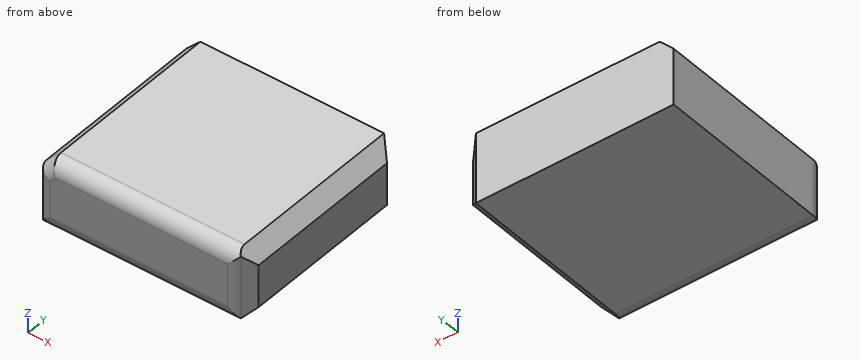
```python
from build123d import *

# Parameters (mm, degrees)
F0_W        = 76.2943662703
F0_H        = 68.5328170657
F1_DEPTH    = 25.4
F2_SIZE     = 5.08
F3_T1_DEPTH = 45.72
F3_T3_DEPTH = 32.5842048969
F3_T5_DEPTH = 96.6143662703
F3_T7_DEPTH = 91.5343662703
F3_T9_DEPTH = 35.9210244843


# Not quite as in the source:
# - a fillet or chamfer that OpenCascade refuses, or shapes differently, is made with other operations: its cross-section is extruded or revolved along the edge and cut away or added


with BuildPart() as f1:
    # F0 (on Top) → F1 (new body)
    with BuildSketch(Plane.XY):
        with Locations((-1.9816737622, 2.3119486868)):
            Rectangle(F0_W, F0_H)
    extrude(amount=F1_DEPTH)

    # F2
    f2_edges = [f1.edges().sort_by_distance(p)[0] for p in [
        (36.165509, -31.95446, 12.7),
        (36.165509, 36.578357, 12.7),
        (36.165509, 2.311949, 0),
        (36.165509, 2.311949, 25.4),
        (-40.128857, 2.311949, 25.4),
    ]]
    chamfer(f2_edges, length=F2_SIZE)

    # F3: fillet of radius 5.08 on 5 edges, made by hand

    # F3_s2 → F3_t1 (cut)
    with BuildSketch(Plane.XY.offset(-12.7)):
        with BuildLine():
            ThreePointArc((-40.1288568974, -26.874459846), (-38.6409593458, -30.4665622944), (-35.0488568974, -31.954459846))
            Line((-35.0488568974, -31.954459846), (-40.1288568974, -31.954459846))
            Line((-40.1288568974, -31.954459846), (-40.1288568974, -26.874459846))
        make_face()
    extrude(amount=F3_T1_DEPTH, mode=Mode.SUBTRACT)

    # F3_s4 → F3_t3 (cut)
    with BuildSketch(Plane(origin=(-18.8846845697, 0, -18.8846845697), x_dir=(0, 1, 0), z_dir=(0.7071067812, 0, 0.7071067812))):
        with BuildLine():
            ThreePointArc((-26.874459846, 42.7437966271), (-30.4665622944, 41.2558990755), (-31.954459846, 37.6637966271))
            Line((-31.954459846, 37.6637966271), (-31.954459846, 42.7437966271))
            Line((-31.954459846, 42.7437966271), (-26.874459846, 42.7437966271))
        make_face()
    extrude(amount=F3_T3_DEPTH, mode=Mode.SUBTRACT)

    # F3_s6 → F3_t5 (cut)
    with BuildSketch(Plane.YZ.offset(-52.8288568974)):
        with BuildLine():
            ThreePointArc((-26.874459846, 0), (-30.4665622944, 1.4878975516), (-31.954459846, 5.08))
            Line((-31.954459846, 5.08), (-31.954459846, 0))
            Line((-31.954459846, 0), (-26.874459846, 0))
        make_face()
    extrude(amount=F3_T5_DEPTH, mode=Mode.SUBTRACT)

    # F3_s8 → F3_t7 (cut)
    with BuildSketch(Plane.YZ.offset(-47.7488568974)):
        with BuildLine():
            ThreePointArc((-26.874459846, 25.4), (-30.4665622944, 23.9121024484), (-31.954459846, 20.32))
            Line((-31.954459846, 20.32), (-31.954459846, 25.4))
            Line((-31.954459846, 25.4), (-26.874459846, 25.4))
        make_face()
    extrude(amount=F3_T7_DEPTH, mode=Mode.SUBTRACT)

    # F3_s10 → F3_t9 (cut)
    with BuildSketch(Plane.XY.offset(-5.2605122421)):
        with BuildLine():
            ThreePointArc((28.9813044761, -31.954459846), (30.9253363125, -31.5677678712), (32.5734069245, -30.4665622944))
            Line((32.5734069245, -30.4665622944), (31.0855093729, -31.954459846))
            Line((31.0855093729, -31.954459846), (28.9813044761, -31.954459846))
        make_face()
    extrude(amount=F3_T9_DEPTH, mode=Mode.SUBTRACT)


solid = f1.part
```
Model file for the job. Use its own axes, mm. Give positions to 0.01 mm unless a question says otherwise; leave off trailing zeros. Order: outer loops, then holes, each group sorted by start corner. A loop starts at its lowest first (then second) coordinate and runs counter-clockwise, first axis right, second up.
1) Pin check, flat tip, straight feed: pin 1 (10 mm diameter, centred on x = 25.5, z = 22, fed in from -Y). Stop position of the tip, or through.
2) Wall check: probe 1 along Y at (x, z) = (21.5, 1.5); probe 2 along X at (y, z) = (9.5, 22.75); probe 3 along X at (y, z) = (15, 3). Give the ranges that are in metal, low to high.
3) Saw through at A-A, the plane y = 19. Write the cut outline in (x, z), then the cut area to 3 significant figures.
4) Saw through at B-B, the plane z = 2.75. Write the cut outline in (x, y).
Computed:
1. pin 1: stops at y = -31.95
2. probe 1: y = -30.48 to 36.58
2. probe 2: x = -37.7 to 33.74
2. probe 3: x = -40.13 to 34.09
3. outline: (-40.13, 0) - (31.09, 0) - (36.17, 5.08) - (36.17, 20.32) - (31.09, 25.4) - (-35.05, 25.4) - (-40.13, 20.32) - close
3. area: 1,900 mm2
4. outline: (-40.13, -26.87) arc R5.08 ccw to (-37.38, -31.39) - (31.31, -31.39) arc R5.08 ccw to (32.57, -30.47) - (33.84, -29.2) - (33.84, 33.83) - (31.09, 36.58) - (-40.13, 36.58) - close
